Verification items for the finished model (mm, model axes). Face numbers are marked on the shaded views. A direction names the side the tool comes from. Give positions to 0.01 mm unless a question says otherwise; leave off trailing zeros. Loops run counter-clockwise (first coordinate to the right, second up) from the corner with the lowest first, then second, coordinate; pieces in that order, holes last. Notation, with made-up numbers: (38, -22.5) - (46, -22.5) arc R13 cw to (46, -9.5) - close; hole circle Ø8 at (-27, 6.25). An arc over 180 degrees is marked (long way). One line per question, with ' | ' between items. Start each with the question number.
1. Section check D-D, the plane y = -85. Enter the section's corners in (x, z).
2. Section check A-A, the plane x = 0. Enter the section's corners in (y, z).
3. Depth check by flat-ended pin: pin 1 Ø10 at (y, z) = (56, 3.5) entering from +X; pin 2 Ø14.5 at (x, y) = (-73.61, 42.5) entering from +Z; pin 3 Ø4 at (x, z) = (-64, 14.5) entering from -Y. Enter the tip coordinate at first touch or a pass-through.
4. Section check B-B, the plane y = 0. Enter the section's corners in (x, z).
5. Section check C-C, the plane z = 11.5. Enter the section's corners in (x, y).
6. Thickness scan on line 1 along Y through (x, z) = (0, 9.75); line 2 along Z through (x, y) = (18, -67); line 3 along Y through (x, z) = (1.5, 14.5). Record the ranges inside material, lowest first. Write a range as from..to.
7. Tool access check on the marked faces 1 and 2. Record the directions out of +Z, -Z, +X, -X, +Y, -Y that give a thin tool (end or side, any length) a straight path to the whole face; none if there is none.
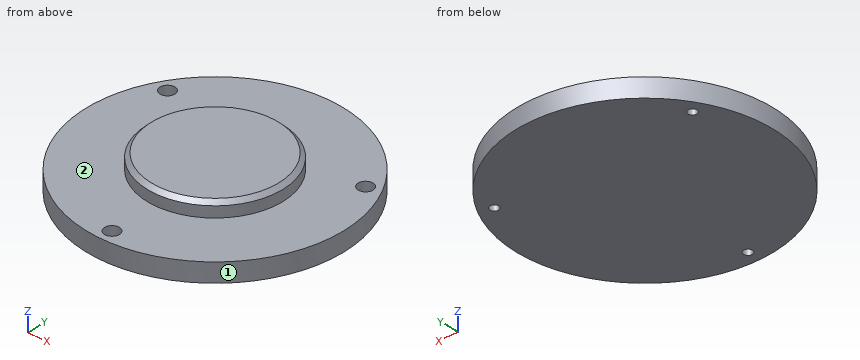
from build123d import *

# Parameters (mm, degrees)
F0_R     = 95
F1_DEPTH = 14
F2_R     = 50
F3_DEPTH = 11
F4_SIZE  = 3
F5_R     = 5.5
F6_DEPTH = 7
F7_R     = 3.25
F8_DEPTH = 25


with BuildPart() as f1:
    # F0 (on Top) → F1 (new body)
    with BuildSketch(Plane.XY):
        Circle(F0_R)
    extrude(amount=F1_DEPTH)

    # F2 (on face) → F3 (join)
    with BuildSketch(Plane.XY.offset(14)):
        Circle(F2_R)
    extrude(amount=F3_DEPTH)

    # F4
    f4_edges = [f1.edges().sort_by_distance(p)[0] for p in [
        (-50, 0, 25),
    ]]
    chamfer(f4_edges, length=F4_SIZE)

    # F5 (on face) → F6 (cut)
    with BuildSketch(Plane.XY.offset(14)):
        with Locations((0, -85)):
            Circle(F5_R)
        with Locations((-73.612159, 42.5)):
            Circle(F5_R)
        with Locations((73.612159, 42.5)):
            Circle(F5_R)
    extrude(amount=-F6_DEPTH, mode=Mode.SUBTRACT)

    # F7 (on face) → F8 (cut)
    with BuildSketch(Plane.XY.offset(7)):
        with Locations((0, -85)):
            Circle(F7_R)
        with Locations((73.612159, 42.5)):
            Circle(F7_R)
        with Locations((-73.612159, 42.5)):
            Circle(F7_R)
    extrude(amount=-F8_DEPTH, mode=Mode.SUBTRACT)


solid = f1.part
Results list:
1) outline: (-42.43, 0) - (-3.25, 0) - (-3.25, 7) - (-5.5, 7) - (-5.5, 14) - (-42.43, 14) - close; (3.25, 0) - (42.43, 0) - (42.43, 14) - (5.5, 14) - (5.5, 7) - (3.25, 7) - close
2) outline: (-95, 0) - (-88.25, 0) - (-88.25, 7) - (-90.5, 7) - (-90.5, 14) - (-95, 14) - close; (-81.75, 0) - (95, 0) - (95, 14) - (50, 14) - (50, 22) - (47, 25) - (-47, 25) - (-50, 22) - (-50, 14) - (-79.5, 14) - (-79.5, 7) - (-81.75, 7) - close
3) pin 1: x = 80.15 | pin 2: z = 14 | pin 3: y = -71.92
4) outline: (-95, 0) - (95, 0) - (95, 14) - (50, 14) - (50, 22) - (47, 25) - (-47, 25) - (-50, 22) - (-50, 14) - (-95, 14) - close
5) outline: circle Ø190 at (0, 0); hole circle Ø11 at (-73.61, 42.5); hole circle Ø11 at (0, -85); hole circle Ø11 at (73.61, 42.5)
6) line 1: -95..-90.5, -79.5..95 | line 2: 0..14 | line 3: -49.98..49.98
7) face 1: +Z, -Z | face 2: +Z
